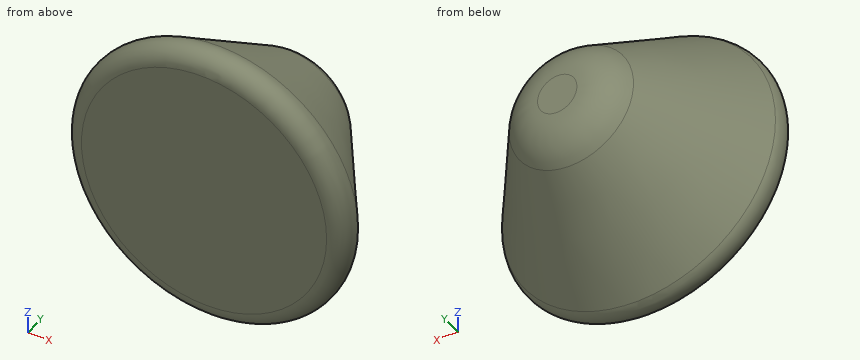
from build123d import *

# Parameters (mm, degrees)
SKETCH3_R           = 9
BOSS_EXTRUDE3_DEPTH = 9
BOSS_EXTRUDE3_TAPER = 35
FILLET1_R           = 3
FILLET2_R           = 1


with BuildPart() as part:
    # Sketch3 → Boss-Extrude3 (new body)
    with BuildSketch(Plane(origin=(0, 0, 0), x_dir=(1, 0, 0), z_dir=(0, 1, 0))):
        Circle(SKETCH3_R)
    extrude(amount=BOSS_EXTRUDE3_DEPTH, taper=BOSS_EXTRUDE3_TAPER)

    # Fillet1
    fillet1_edges = [part.edges().sort_by_distance(p)[0] for p in [
        (-2.698132156, 9, 0),
    ]]
    fillet(fillet1_edges, radius=FILLET1_R)

    # Fillet2
    fillet2_edges = [part.edges().sort_by_distance(p)[0] for p in [
        (-9, 0, 0),
    ]]
    fillet(fillet2_edges, radius=FILLET2_R)


solid = part.part
Part model, mm, in its own coordinate system. Coordinates: 2 decimals unless noted, no trailing zeros. Loops run counter-clockwise (first coordinate to the right, second up) from the corner with the lowest first, then second, coordinate; pieces in that order, holes last. Notation, with made-up numbers: M 38.25,40 L 73.25,40 A14 ccw 73.25,46 Z; hole C -35,-20 d5. An arc over 180 degrees is marked long. Use a Markdown table: item, result. Add a question column.
Q1. Probe L1, parallel to Z at x = 4.5, y = 4.5; L2, parallel to Y at x = -3.5, z = -6; L3, parallel to Y at x = 3, z = -4.5. List the from-to ranges inside material, lowest first.
Q2. Cut at A-A (y = 6.5). Write the cut outline in (x, z), and give its area (3 significant figures).
Q3. Pin check, flat tips, straight feed: P1, Ø2, axis at x = 1, y = 2.5, coming from the +Z side; P2, Ø4, axis at y = 3, z = 5.5, coming from the -X side; P3, Ø5, axis at x = 0.5, y = 7, coming from the +Z side; P4, Ø8, axis at x = 1.5, z = 0, coming from the +Y side. Stop position of each tip, or through.
Q4. Cut at B-B (y = 4.5). Write the cut outline in (x, z), and give its area (3 significant figures).
Worked out:
| question | item | result |
|---|---|---|
| 1 | L1 | z = -3.74 to 3.74 |
| 1 | L2 | y = 0 to 2.93 |
| 1 | L3 | y = 0 to 5.13 |
| 2 | outline | C 0,0 d8.9 |
| 2 | area | 62.2 mm2 |
| 3 | P1 | stops at z = 7.89 |
| 3 | P2 | stops at x = -6.76 |
| 3 | P3 | stops at z = 5.84 |
| 3 | P4 | stops at y = 9 |
| 4 | outline | C 0,0 d11.7 |
| 4 | area | 107 mm2 |
